Design review of the part built by this model. Coordinates are the model's own, in mm. A direction names the side the tool comes from. Round coordinates to 2 decimals unless told otherwise and drop trailing zeros. Loops run counter-clockwise (first coordinate to the right, second up) from the corner with the lowest first, then second, coordinate; pieces in that order, holes last. Notation, with made-up numbers: M 52.25,54 L 58.25,54 A22 ccw 58.25,69 Z; hole C -40,76.5 d7. An arc over 180 degrees is marked long. One line per item, written item: value. Start each with the question number.
Item 1: For faces 1 (the flat face through (0, 0, 0)), 2 (the flat face through (9, 12, 15.647)), 3 (the flat face through (1.05, 11, 21)), list the 3-axis set-ups (+Z, -Z, +X, -X, +Y, -Y) from which the entire face can be reached by the end or side of a thin tool; tool diameter is ignored.
Item 2: We need section B-B (x = 0). Write out the cut boundary in (y, z), then the cut area to 3 significant figures.
Item 3: We need section C-C (z = -14). Write out the cut boundary in (x, y), then the cut area to 3 significant figures.
Item 4: We need section D-D (z = -8.5). Write out the cut boundary in (x, y).
Item 5: Mouldability with a two-part tool opening along Z and no side actions: class faces 4 (the flat face through (0, 9, 17.2)), 5 (the flat face through (12.15, 11, 22)), 6 (the flat face through (-9.25, 12, 14)), 7 (the flat face through (0, 11, 20.7)) as released by +Z, released by -Z, zero draft, split by the parting line, or undercut.
Item 6: Clearance check with flat-ended pins moving along their axes: pin 1 (0.5 mm diameter, centred on x = 16, y = 21.5, fed in from -Z); pin 2 (0.8 mm diameter, centred on x = -16.5, y = 21.5, fed in from -Z); pin 3 (14.5 mm diameter, centred on x = 6.5, z = 3, fed in from +Y). State where each tip first meets the part, or that it passes through.
Item 7: We need section A-A (y = 16.5). Write out the cut boundary in (x, z), then the cut area to 3 significant figures.
Item 8: For line 1 along X through (y, z) = (19.9, 0); line 2 along Y through (x, z) = (6, -3); line 3 along Z through (x, y) = (0, 13.5), list the stretches that pass through material, from the lowest coordinate up.
from build123d import *

# Parameters (mm, degrees)
BOSS_EXTRUDE12_DEPTH = 22
SKETCH1_14_R         = 2
BOSS_EXTRUDE13_DEPTH = 21
BOSS_EXTRUDE14_DEPTH = 3
SKETCH1_16_W         = 16.2
SKETCH1_16_H         = 1.552983906
BOSS_EXTRUDE15_DEPTH = 3
SKETCH1_17_W         = 16.2
SKETCH1_17_H         = 3.844417312
BOSS_EXTRUDE16_DEPTH = 15
SKETCH1_18_R         = 2
BOSS_EXTRUDE17_DEPTH = 18
SKETCH1_19_W         = 4.05
SKETCH1_19_H         = 1.155582688
BOSS_EXTRUDE18_DEPTH = 22
SKETCH1_20_W         = 16.2
SKETCH1_20_H         = 1.155582688
BOSS_EXTRUDE19_DEPTH = 15
SKETCH10_R           = 2
CUT_EXTRUDE6_DEPTH   = 3
SKETCH10_10_W        = 2.1
SKETCH10_10_H        = 2.1
CUT_EXTRUDE7_DEPTH   = 1.5
BOSS_EXTRUDE20_DEPTH = 3


with BuildPart() as part:
    # Sketch1 → Boss-Extrude12 (new body)
    with BuildSketch(Plane(origin=(0, 0, 0), x_dir=(1, 0, 0), z_dir=(0, 1, 0))):
        with BuildLine():
            ThreePointArc((-17.7, -3.6), (-21.3, 0), (-17.7, 3.6))
            Line((-17.7, 3.6), (-14.149204925, 3.6))
            ThreePointArc((-14.149204925, 3.6), (0, 14.6), (14.149204925, 3.6))
            Line((14.149204925, 3.6), (17.7, 3.6))
            ThreePointArc((17.7, 3.6), (21.3, 0), (17.7, -3.6))
            Line((17.7, -3.6), (14.149204925, -3.6))
            ThreePointArc((14.149204925, -3.6), (12.316145556, -7.840443778), (9.25, -11.295906338))
            Line((9.25, -11.295906338), (9.25, -15.647016094))
            Line((9.25, -15.647016094), (8.1, -15.647016094))
            Line((8.1, -15.647016094), (8.1, -17.2))
            Line((8.1, -17.2), (8.1, -21.044417312))
            Line((8.1, -21.044417312), (12.15, -21.044417312))
            Line((12.15, -21.044417312), (24.3, 0))
            Line((24.3, 0), (12.15, 21.044417312))
            Line((12.15, 21.044417312), (-12.15, 21.044417312))
            Line((-12.15, 21.044417312), (-24.3, 0))
            Line((-24.3, 0), (-12.15, -21.044417312))
            Line((-12.15, -21.044417312), (-8.1, -21.044417312))
            Line((-8.1, -21.044417312), (-8.1, -17.2))
            Line((-8.1, -17.2), (-8.1, -15.647016094))
            Line((-8.1, -15.647016094), (-9.25, -15.647016094))
            Line((-9.25, -15.647016094), (-9.25, -11.295906338))
            ThreePointArc((-9.25, -11.295906338), (-12.316145556, -7.840443778), (-14.149204925, -3.6))
            Line((-14.149204925, -3.6), (-17.7, -3.6))
        make_face()
    extrude(amount=BOSS_EXTRUDE12_DEPTH)

    # Sketch1_14 → Boss-Extrude13 (add)
    # profile 1 of 2: a face of its own
    with BuildSketch(Plane(origin=(0, 0, 0), x_dir=(1, 0, 0), z_dir=(0, 1, 0))):
        with BuildLine():
            Line((17.7, 3.6), (14.149204925, 3.6))
            ThreePointArc((14.149204925, 3.6), (14.6, 0), (14.149204925, -3.6))
            Line((14.149204925, -3.6), (17.7, -3.6))
            ThreePointArc((17.7, -3.6), (21.3, 0), (17.7, 3.6))
        make_face()
        with Locations(Location((17.5, 0, 0), (0, 0, 90))):
            Circle(SKETCH1_14_R, mode=Mode.SUBTRACT)
    # profile 2 of 2: a face of its own
    with BuildSketch(Plane(origin=(0, 0, 0), x_dir=(1, 0, 0), z_dir=(0, 1, 0))):
        with BuildLine():
            Line((-14.149204925, 3.6), (-17.7, 3.6))
            ThreePointArc((-17.7, 3.6), (-21.3, 0), (-17.7, -3.6))
            Line((-17.7, -3.6), (-14.149204925, -3.6))
            ThreePointArc((-14.149204925, -3.6), (-14.6, 0), (-14.149204925, 3.6))
        make_face()
        with Locations(Location((-17.5, 0, 0), (0, 0, 90))):
            Circle(SKETCH1_14_R, mode=Mode.SUBTRACT)
    extrude(amount=BOSS_EXTRUDE13_DEPTH)

    # Sketch1_15 → Boss-Extrude14 (add)
    with BuildSketch(Plane(origin=(0, 0, 0), x_dir=(1, 0, 0), z_dir=(0, 1, 0))):
        with BuildLine():
            ThreePointArc((14.149204925, 3.6), (0, 14.6), (-14.149204925, 3.6))
            ThreePointArc((-14.149204925, 3.6), (-14.6, 0), (-14.149204925, -3.6))
            ThreePointArc((-14.149204925, -3.6), (-12.316145556, -7.840443778), (-9.25, -11.295906338))
            Line((-9.25, -11.295906338), (-9.25, 0))
            Line((-9.25, 0), (9.25, 0))
            Line((9.25, 0), (9.25, -11.295906338))
            ThreePointArc((9.25, -11.295906338), (12.316145556, -7.840443778), (14.149204925, -3.6))
            ThreePointArc((14.149204925, -3.6), (14.6, 0), (14.149204925, 3.6))
        make_face()
    extrude(amount=BOSS_EXTRUDE14_DEPTH)

    # Sketch1_16 → Boss-Extrude15 (add)
    with BuildSketch(Plane(origin=(0, 0, 0), x_dir=(1, 0, 0), z_dir=(0, 1, 0))):
        with Locations((0, -16.423508047)):
            Rectangle(SKETCH1_16_W, SKETCH1_16_H)
    extrude(amount=BOSS_EXTRUDE15_DEPTH)

    # Sketch1_17 → Boss-Extrude16 (add)
    with BuildSketch(Plane(origin=(0, 0, 0), x_dir=(1, 0, 0), z_dir=(0, 1, 0))):
        with Locations((0, -19.122208656)):
            Rectangle(SKETCH1_17_W, SKETCH1_17_H)
    extrude(amount=BOSS_EXTRUDE16_DEPTH)

    # Sketch1_18 → Boss-Extrude17 (add)
    with BuildSketch(Plane(origin=(0, 0, 0), x_dir=(1, 0, 0), z_dir=(0, 1, 0))):
        with Locations(Location((17.5, 0, 0), (0, 0, 90))):
            Circle(SKETCH1_18_R)
        with Locations(Location((-17.5, 0, 0), (0, 0, 90))):
            Circle(SKETCH1_18_R)
    extrude(amount=BOSS_EXTRUDE17_DEPTH)

    # Sketch1_19 → Boss-Extrude18 (add)
    with BuildSketch(Plane(origin=(0, 0, 0), x_dir=(1, 0, 0), z_dir=(0, 1, 0))):
        with Locations((-10.125, -21.622208656)):
            Rectangle(SKETCH1_19_W, SKETCH1_19_H)
        with Locations((10.125, -21.622208656)):
            Rectangle(SKETCH1_19_W, SKETCH1_19_H)
    extrude(amount=BOSS_EXTRUDE18_DEPTH)

    # Sketch1_20 → Boss-Extrude19 (add)
    with BuildSketch(Plane(origin=(0, 0, 0), x_dir=(1, 0, 0), z_dir=(0, 1, 0))):
        with Locations((0, -21.622208656)):
            Rectangle(SKETCH1_20_W, SKETCH1_20_H)
    extrude(amount=BOSS_EXTRUDE19_DEPTH)

    # Sketch10 → Cut-Extrude6 (cut)
    with BuildSketch(Plane.XY.offset(22.2)):
        with Locations((0, 5)):
            Circle(SKETCH10_R)
    extrude(amount=-CUT_EXTRUDE6_DEPTH, mode=Mode.SUBTRACT)

    # Sketch10_10 → Cut-Extrude7 (cut)
    with BuildSketch(Plane.XY.offset(22.2)):
        with Locations((0, 11.05)):
            Rectangle(SKETCH10_10_W, SKETCH10_10_H)
    extrude(amount=-CUT_EXTRUDE7_DEPTH, mode=Mode.SUBTRACT)

    # Sketch1_21 → Boss-Extrude20 (add)
    with BuildSketch(Plane(origin=(0, 0, 0), x_dir=(1, 0, 0), z_dir=(0, 1, 0))):
        with BuildLine():
            Line((-9.25, 0), (-9.25, -11.295906338))
            ThreePointArc((-9.25, -11.295906338), (-8.685431593, -11.735556146), (-8.1, -12.147016094))
            Line((-8.1, -12.147016094), (-8.1, -15.647016094))
            Line((-8.1, -15.647016094), (8.1, -15.647016094))
            Line((8.1, -15.647016094), (8.1, -12.147016094))
            ThreePointArc((8.1, -12.147016094), (8.685431593, -11.735556146), (9.25, -11.295906338))
            Line((9.25, -11.295906338), (9.25, 0))
            Line((9.25, 0), (-9.25, 0))
        make_face()
        with BuildLine():
            ThreePointArc((-8.1, -12.147016094), (-8.685431593, -11.735556146), (-9.25, -11.295906338))
            Line((-9.25, -11.295906338), (-9.25, -15.647016094))
            Line((-9.25, -15.647016094), (-8.1, -15.647016094))
            Line((-8.1, -15.647016094), (-8.1, -12.147016094))
        make_face()
        with BuildLine():
            Line((9.25, -15.647016094), (9.25, -11.295906338))
            ThreePointArc((9.25, -11.295906338), (8.685431593, -11.735556146), (8.1, -12.147016094))
            Line((8.1, -12.147016094), (8.1, -15.647016094))
            Line((8.1, -15.647016094), (9.25, -15.647016094))
        make_face()
    extrude(amount=BOSS_EXTRUDE20_DEPTH)


solid = part.part
A:
1. face 1: +Z, -Z, +X, -X, -Y
1. face 2: +Y
1. face 3: +Z
2. outline: M 0,-21.04 L 22,-21.04 L 22,-14.6 L 3,-14.6 L 3,17.2 L 15,17.2 L 15,22.2 L 12.1,22.2 L 12.1,20.7 L 10,20.7 L 10,22.2 L 7,22.2 L 7,19.2 L 3,19.2 L 3,22.2 L 0,22.2 Z
2. area: 297 mm2
3. outline: M -16.22,0 L 16.22,0 L 16.22,22 L 4.14,22 L 4.14,3 L -4.14,3 L -4.14,22 L -16.22,22 Z
3. area: 556 mm2
4. outline: M -19.39,0 L 19.39,0 L 19.39,22 L 11.87,22 L 11.87,3 L -11.87,3 L -11.87,22 L -19.39,22 Z
5. face 4: undercut
5. face 5: zero draft
5. face 6: undercut
5. face 7: released by +Z
6. pin 1: z = -14.81
6. pin 2: z = -14.2
6. pin 3: y = 3
7. outline: M -24.3,0 L -12.15,-21.04 L 12.15,-21.04 L 24.3,0 L 12.15,21.04 L 12.15,22.2 L 8.1,22.2 L 8.1,15.65 L 9.25,15.65 L 9.25,11.3 A14.6 cw long -9.25,11.3 L -9.25,15.65 L -8.1,15.65 L -8.1,22.2 L -12.15,22.2 L -12.15,21.04 Z
7. area: 748 mm2
8. line 1: -24.3 to -19.5, -15.5 to -14.6, 14.6 to 15.5, 19.5 to 24.3
8. line 2: 0 to 3
8. line 3: -21.04 to -14.6, 17.2 to 22.2
